from build123d import *

# Parameters (mm, degrees)
SKETCH1_W           = 63.5
SKETCH1_H           = 19.05
BOSS_EXTRUDE1_DEPTH = 6.35
SKETCH2_W           = 30.48
SKETCH2_H           = 19.05
BOSS_EXTRUDE2_DEPTH = 26.67
CUT_EXTRUDE1_REACH  = 8.35
SKETCH3_R           = 3.302
SKETCH4_R           = 12.669104941
CUT_EXTRUDE2_DEPTH  = 8.89
SKETCH5_R           = 3.302
CUT_EXTRUDE3_DEPTH  = 20.05
FILLET1_R           = 12.7


with BuildPart() as part:
    # Sketch1 → Boss-Extrude1 (new body)
    with BuildSketch(Plane(origin=(0, 0, 0), x_dir=(1, 0, 0), z_dir=(0, 1, 0))):
        with Locations((-30.537406907, 4.286893637)):
            Rectangle(SKETCH1_W, SKETCH1_H)
    extrude(amount=BOSS_EXTRUDE1_DEPTH)

    # Sketch2 → Boss-Extrude2 (add)
    with BuildSketch(Plane(origin=(0, 6.35, 0), x_dir=(1, 0, 0), z_dir=(0, 1, 0))):
        with Locations((-30.537406907, 4.286893637)):
            Rectangle(SKETCH2_W, SKETCH2_H)
    extrude(amount=BOSS_EXTRUDE2_DEPTH)

    # Sketch3 → Cut-Extrude1 (cut, up to next)
    with BuildSketch(Plane(origin=(0, 6.35, 0), x_dir=(1, 0, 0), z_dir=(0, 1, 0)), mode=Mode.PRIVATE) as cut_extrude1_sk1:
        with Locations((-54.032406907, 4.286893637)):
            Circle(SKETCH3_R)
    cut_extrude1_tool1 = extrude(cut_extrude1_sk1.sketch, amount=-CUT_EXTRUDE1_REACH, mode=Mode.PRIVATE) & part.part
    add(cut_extrude1_tool1.solids().sort_by_distance((-54.032407, 6.35, -4.286894))[0], mode=Mode.SUBTRACT)
    # Sketch3 → Cut-Extrude1 (cut, up to next)
    with BuildSketch(Plane(origin=(0, 6.35, 0), x_dir=(1, 0, 0), z_dir=(0, 1, 0)), mode=Mode.PRIVATE) as cut_extrude1_sk2:
        with Locations((-7.042406907, 4.286893637)):
            Circle(SKETCH3_R)
    cut_extrude1_tool2 = extrude(cut_extrude1_sk2.sketch, amount=-CUT_EXTRUDE1_REACH, mode=Mode.PRIVATE) & part.part
    add(cut_extrude1_tool2.solids().sort_by_distance((-7.042407, 6.35, -4.286894))[0], mode=Mode.SUBTRACT)

    # Sketch4 → Cut-Extrude2 (cut)
    with BuildSketch(Plane.XY.offset(5.238106363)):
        with Locations((-30.537406907, 18.034)):
            Circle(SKETCH4_R)
    extrude(amount=-CUT_EXTRUDE2_DEPTH, mode=Mode.SUBTRACT)

    # Sketch5 → Cut-Extrude3 (cut, through all)
    with BuildSketch(Plane.XY.offset(5.238106363)):
        with Locations((-30.537406907, 18.034)):
            Circle(SKETCH5_R)
    extrude(amount=-CUT_EXTRUDE3_DEPTH, mode=Mode.SUBTRACT)

    # Fillet1
    fillet1_edges = [part.edges().sort_by_distance(p)[0] for p in [
        (-45.777406907, 33.02, -4.286893637),
        (-15.297406907, 33.02, -4.286893637),
    ]]
    fillet(fillet1_edges, radius=FILLET1_R)


solid = part.part
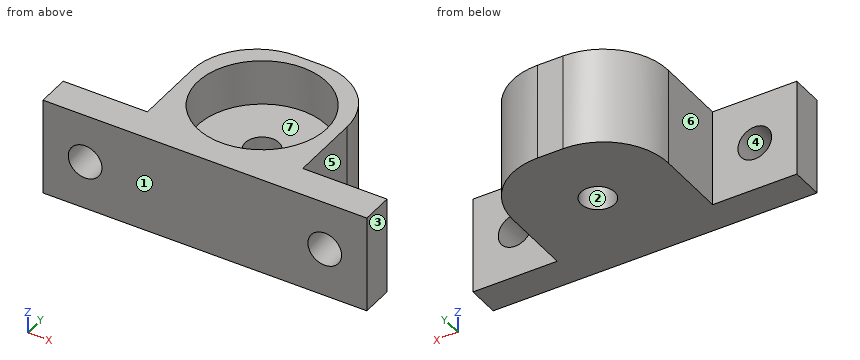
Check sheet for the modelled part. Datum: model origin and axes. Units: mm. Face numbers are marked on the shaded views. A direction names the side the tool comes from. Give positions to 0.01 mm unless a question says otherwise; leave off trailing zeros. Loops run counter-clockwise (first coordinate to the right, second up) from the corner with the lowest first, then second, coordinate; pieces in that order, holes last. Notation, with made-up numbers: M 48,-26 L 52,-26 A17 cw 52,-10 Z; hole C -35.5,60.25 d7. An arc over 180 degrees is marked long. Answer as a JSON object with one key per item and string values. Group by question number.
Q1. Release check for a two-part mould opening along X. For the marked faces 1, 2 and 3 record: released by +X, released by -X, zero draft, split by the parting line, or undercut.
Q2. Cross-section at B-B on x = -52. Record the cut outline in (y, z), then the cut area to 3 significant figures.
Q3. Material ranges on line 1 along Z through (x, y) = (-18.5, 20); line 2 along X through (y, z) = (12.5, -4); line 3 along X through (y, z) = (20, -3.75), recorded low to high. Write a range as [from, to].
Q4. Go/stop test with flat-tipped pins: P1, Ø1.5, axis at x = -42.5, z = 2.5, coming from the +Y side; P2, Ø10, axis at y = 13, z = -8.5, coming from the -X side; P3, Ø5, axis at x = -53, z = -6.5, coming from the +Y side. Record where each tip stops, or that it passes through.
Q5. Cross-section at D-D on z = -11. Record the cut outline in (x, y).
Q6. Access from +Z, -Z, +X, -X, +Y, -Y to the whole of each face (thin tool, end or side, straight path). Record for the marked faces 4, 5, 6 and 7.
Q7. Cross-section at C-C on y = 29. Record the cut outline in (x, z), then the cut area to 3 significant figures.
Q8. Cross-section at A-A on z = -5. Record the cut outline in (x, y).
Evaluation:
{
 "1": {"face 1": "zero draft", "face 2": "undercut", "face 3": "released by +X"},
 "2": {"outline": "M 0,-13.81 L 6.35,-13.81 L 6.35,-6.89 L 0,-6.89 Z; M 0,-1.68 L 6.35,-1.68 L 6.35,5.24 L 0,5.24 Z", "area": "87.9 mm2"},
 "3": {"line 1": "z = [-13.81, -3.65]", "line 2": "x = [-45.78, -15.3]", "line 3": "x = [-45.78, -33.19], [-27.88, -15.3]"},
 "4": {"P1": "stops at y = 29.6", "P2": "stops at x = -45.78", "P3": "stops at y = 6.35"},
 "5": {"outline": "M -62.29,0 L 1.21,0 L 1.21,6.35 L -15.3,6.35 L -15.3,20.32 A12.7 ccw -28,33.02 L -33.08,33.02 A12.7 ccw -45.78,20.32 L -45.78,6.35 L -62.29,6.35 Z; hole C -30.54,18.03 d6.6"},
 "6": {"face 4": "+Y, -Y", "face 5": "+Z, -Z, +X, +Y", "face 6": "+Z, -Z, -X, +Y", "face 7": "+Z"},
 "7": {"outline": "M -42.35,-13.81 L -18.73,-13.81 L -18.73,5.24 L -24.19,5.24 L -24.19,-3.65 L -36.88,-3.65 L -36.88,5.24 L -42.35,5.24 Z", "area": "337 mm2"},
 "8": {"outline": "M -62.29,0 L -57.26,0 L -57.26,6.35 L -62.29,6.35 Z; M -50.81,0 L -10.27,0 L -10.27,6.35 L -15.3,6.35 L -15.3,20.32 A12.7 ccw -28,33.02 L -33.08,33.02 A12.7 ccw -45.78,20.32 L -45.78,6.35 L -50.81,6.35 Z; M -3.82,0 L 1.21,0 L 1.21,6.35 L -3.82,6.35 Z; hole C -30.54,18.03 d6.6"}
}
